CAD build for the part. Positions are in the model's coordinates, mm. A direction names the side the tool comes from. Give positions to 0.01 mm unless a question says otherwise; leave off trailing zeros. Write each loop counter-clockwise with the first axis right and the second up, starting at its lowest first coordinate (ties: lowest second). Pieces come first, ordered by that corner, then holes. Notation, with made-up numbers: (0, 37.5) - (28, 37.5) arc R9 ccw to (28, 54.5) - close; hole circle Ø5 at (10.25, 0.5). An arc over 180 degrees is marked (long way). Answer as a JSON object with one key per item and string values.
Autodesk Inventor part; units mm, degrees
ref_plane "YZ Plane" through (0, 0, 0) normal (1, 0, 0) x (0, 1, 0)
ref_plane "XZ Plane" through (0, 0, 0) normal (0, 1, 0) x (-1, 0, 0)
ref_plane "XY Plane" through (0, 0, 0) normal (0, 0, 1) x (1, 0, 0)
sketch "Boceto1" plane through (0, 0, 0) normal (1, 0, 0) x (0, 1, 0)
  circle A0 centre (0, 0) radius 2.9
  line L0 (2.2, 1.8894) -> (2.2, -1.8894)
  line L1 (-2.2, 1.8894) -> (-2.2, -1.8894)
  circle A1 centre (0, 0) radius 6.5
  dimension "d0" = 5.8
  dimension "d1" = 2.2
  dimension "d2" = 2.2
  dimension "d3" = 13
extrude "Extrusión1" add sketch "Boceto1" along normal blind 9 contours A0 L0 | L1 A0 | A1
sketch "Boceto2" plane through (9, 0, 0) normal (1, 0, 0) x (0, 0, -1)
  circle A0 centre (0, 0) radius 6.5
  line L0 (3.2, -3.2) -> (-3.2, -3.2)
  line L1 (-3.2, -3.2) -> (-3.2, 3.2)
  line L2 (-3.2, 3.2) -> (3.2, 3.2)
  line L3 (3.2, 3.2) -> (3.2, -3.2)
  line L4 (3.2, -3.2) -> (-3.2, 3.2) construction
  line L5 (-3.2, -3.2) -> (3.2, 3.2) construction
  dimension "d6" = 6.4
  dimension "d7" = 6.4
extrude "Extrusión2" add sketch "Boceto2" along normal blind 10
properties part number "Adaptador"
Item 1: Cut at D-D (z = 2.5). Give the cut face in (x, y).
Entries:
{"outline": "(0, -6) - (19, -6) - (19, -3.2) - (9, -3.2) - (9, -1.47) - (0, -1.47) - close; (0, 1.47) - (9, 1.47) - (9, 3.2) - (19, 3.2) - (19, 6) - (0, 6) - close"}
Item 2: Mould opens along Z. For faces 4 (the flat face through (9, -1, 3)), 5 (the cylindrical face through (7.26, 3.07, -5.73)), 6 (the flat face through (19, 0, -4)) say: +Z half, -Z half, draft (parallel to the pull), parting line (faces both ways), or undercut.
Entries:
{"face 4": "undercut", "face 5": "parting line", "face 6": "draft"}
Item 3: Cut at A-A (z = 0.25). Give the cut face in (x, y).
Entries:
{"outline": "(0, -6.5) - (19, -6.5) - (19, -3.2) - (9, -3.2) - (9, -2.2) - (0, -2.2) - close; (0, 2.2) - (9, 2.2) - (9, 3.2) - (19, 3.2) - (19, 6.5) - (0, 6.5) - close"}
Item 4: Probe line 1 (Z direction, x = 13, y = 0.25); line 2 (Y direction, x = 3.5, z = -0.5); line 3 (X direction, y = -2.5, z = 0). List the from-to ranges inside material, lowest first. Write a range as from..to.
Entries:
{"line 1": "-6.5..-3.2, 3.2..6.5", "line 2": "-6.48..-2.2, 2.2..6.48", "line 3": "0..9"}
Item 5: Flat gauge pins, fed straight in: P1, Ø2, axis at x = 3.5, z = -4.5, coming from the +Y side; P2, Ø3, axis at x = 6.5, z = 1.5, coming from the +Y side; P3, Ø3, axis at y = 0.5, z = 0.5, coming from the +X side; P4, Ø4, axis at x = 4, z = -2.5, coming from the -Y side. Where does each tip first touch, or does it go through?
Entries:
{"P1": "y = 5.48", "P2": "y = 6.5", "P3": "through", "P4": "y = -6.48"}
Item 6: Which spindle directions (+Z, -Z, +X, -X, +Y, -Y) get a long thin tool onto all of the face, cutting with end or side? Do faces 1 (the flat face through (0, 3, 0)), 2 (the flat face through (14, 0, 3.2)), 3 (the cylindrical face through (4.4, 0, 2.9)). Say none if no direction does.
Entries:
{"face 1": "+Z, -Z, -X, +Y, -Y", "face 2": "+X", "face 3": "+X, -X"}
Item 7: Cut at B-B (x = 4). Give the cut face in (y, z), and give its area (3 significant figures).
Entries:
{"outline": "circle Ø13 at (0, 0); hole (-2.2, -1.89) arc R2.9 ccw to (2.2, -1.89) - (2.2, 1.89) arc R2.9 ccw to (-2.2, 1.89) - close", "area": "110 mm2"}
